from build123d import *

# Parameters (mm, degrees)
SKETCH_2_R          = 1.5
CUT_EXTRUDE_1_DEPTH = 10


with BuildPart() as part:
    # Эскиз1 → Повернуть1 (revolve)
    with BuildSketch(Plane.XY):
        Polygon((8, 19.5), (4, 19.5), (4, 0), (8, 0), (8, 7.5), (6.365, 7.5), (6.365, 18.5), (8, 18.5), align=None)
    revolve(axis=Axis((0, -1000, 0), (0, 1, 0)))

    # Эскиз2 → Вырез-Вытянуть1 (cut)
    with BuildSketch(Plane.XY):
        with Locations((0, 3.5)):
            Circle(SKETCH_2_R)
    extrude(amount=-CUT_EXTRUDE_1_DEPTH, mode=Mode.SUBTRACT)


solid = part.part
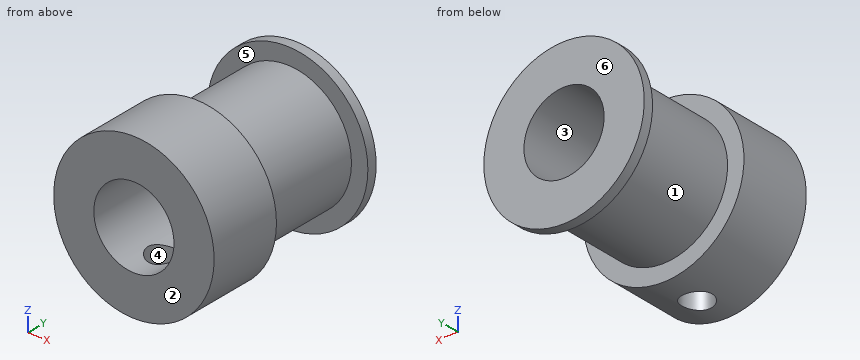
Could you check a few things on this model? Use its own coordinates, in mm. Face numbers are marked on the shaded views. A direction names the side the tool comes from. Round coordinates to 2 decimals unless told otherwise and drop trailing zeros. Write each loop counter-clockwise with the first axis right and the second up, starting at its lowest first coordinate (ties: lowest second). Pieces come first, ordered by that corner, then holes. Notation, with made-up numbers: (86.5, 55.25) - (122.5, 55.25) arc R30 cw to (122.5, 88.25) - close; hole circle Ø4 at (80.5, 39). An arc over 180 degrees is marked (long way). Put each result on its own line as item: value. Start each with the question number.
(1) Thinking about a two-plate mould opening in Z: for the marked faces 1, 2 and 3, which applies, released by +Z, released by -Z, zero draft, split by the parting line, or undercut?
(2) I want a section at A-A, the plane x = 0. Please give me the cut outline in (y, z) (3 decimals), plus the area to 3 significant figures.
(3) I need wall thicknesses on probe 1 along Y at (x, z) = (0, -6.4); probe 2 along Y at (x, z) = (0, -6.1); probe 3 along X at (y, z) = (15.25, 0) (3 decimals). Which ranges of each line are inside material? Lowest first, please.
(4) I want a section at C-C, the plane y = 1.5. Please give me the cut outline in (x, z), plus the area to 3 significant figures.
(5) Will these pins go through, and if not, where does the flat tip stop? pin 1 (5 mm diameter, centred on x = 0, y = 3.5, fed in from -Z); pin 2 (7 mm diameter, centred on x = 0, z = 0, fed in from +Y); pin 3 (1.5 mm diameter, centred on y = 13.5, z = -4.5, fed in from -X); pin 4 (6 mm diameter, centred on x = 5, y = 7.5, fed in from +Z).
(6) For the marked faces 4, 5 and 6, which set-ups out of +Z, -Z, +X, -X, +Y, -Y let a thin tool reach every point of the face, with its end or its side?
(7) I want a section at D-D, the plane x = -3.25. Please give me the cut outline in (y, z), plus the area to 3 significant figures.
(8) I want a section at B-B, the plane z = -2.5. Please give me the cut outline in (x, y).
Here are the results:
1. face 1: split by the parting line
1. face 2: zero draft
1. face 3: undercut
2. outline: (0, -8) - (2, -8) - (2, -4) - (0, -4) - close; (0, 4) - (19.5, 4) - (19.5, 8) - (18.5, 8) - (18.5, 6.365) - (7.5, 6.365) - (7.5, 8) - (0, 8) - close; (5, -8) - (7.5, -8) - (7.5, -6.365) - (18.5, -6.365) - (18.5, -8) - (19.5, -8) - (19.5, -4) - (5, -4) - close
2. area: 108 mm^2
3. probe 1: y = 0 to 2, 5 to 7.5, 18.5 to 19.5
3. probe 2: y = 0 to 2, 5 to 19.5
3. probe 3: x = -6.365 to -4, 4 to 6.365
4. outline: circle Ø16 at (0, 0); hole circle Ø8 at (0, 0)
4. area: 151 mm^2
5. pin 1: stops at z = -8
5. pin 2: passes through
5. pin 3: stops at x = -5.14
5. pin 4: stops at z = 7.75
6. face 4: -Z
6. face 5: none
6. face 6: +Z, -Z, +X, -X, +Y
7. outline: (0, -7.31) - (7.5, -7.31) - (7.5, -5.47) - (18.5, -5.47) - (18.5, -7.31) - (19.5, -7.31) - (19.5, -2.33) - (0, -2.33) - close; (0, 2.33) - (19.5, 2.33) - (19.5, 7.31) - (18.5, 7.31) - (18.5, 5.47) - (7.5, 5.47) - (7.5, 7.31) - (0, 7.31) - close
7. area: 154 mm^2
8. outline: (-7.6, 0) - (-3.12, 0) - (-3.12, 19.5) - (-7.6, 19.5) - (-7.6, 18.5) - (-5.85, 18.5) - (-5.85, 7.5) - (-7.6, 7.5) - close; (3.12, 0) - (7.6, 0) - (7.6, 7.5) - (5.85, 7.5) - (5.85, 18.5) - (7.6, 18.5) - (7.6, 19.5) - (3.12, 19.5) - close
